Source: three-view drawing plus pictorial views. Frame: mm from the lowest corner of the part. A direction names the side the tool comes from. Coordinates: 2 decimals unless noted, no trailing zeros. Order: outer loops, then holes, each group sorted by start corner. A loop starts at its lowest first (then second) coordinate and runs counter-clockwise, first axis right, second up. Notation, with made-up numbers: (78.25, 55.5) - (136.25, 55.5) arc R23 cw to (136.25, 74.5) - close; hole circle Ø8 at (48, 16). An arc over 180 degrees is marked (long way). Use a Markdown table: item, result. Add a question column.
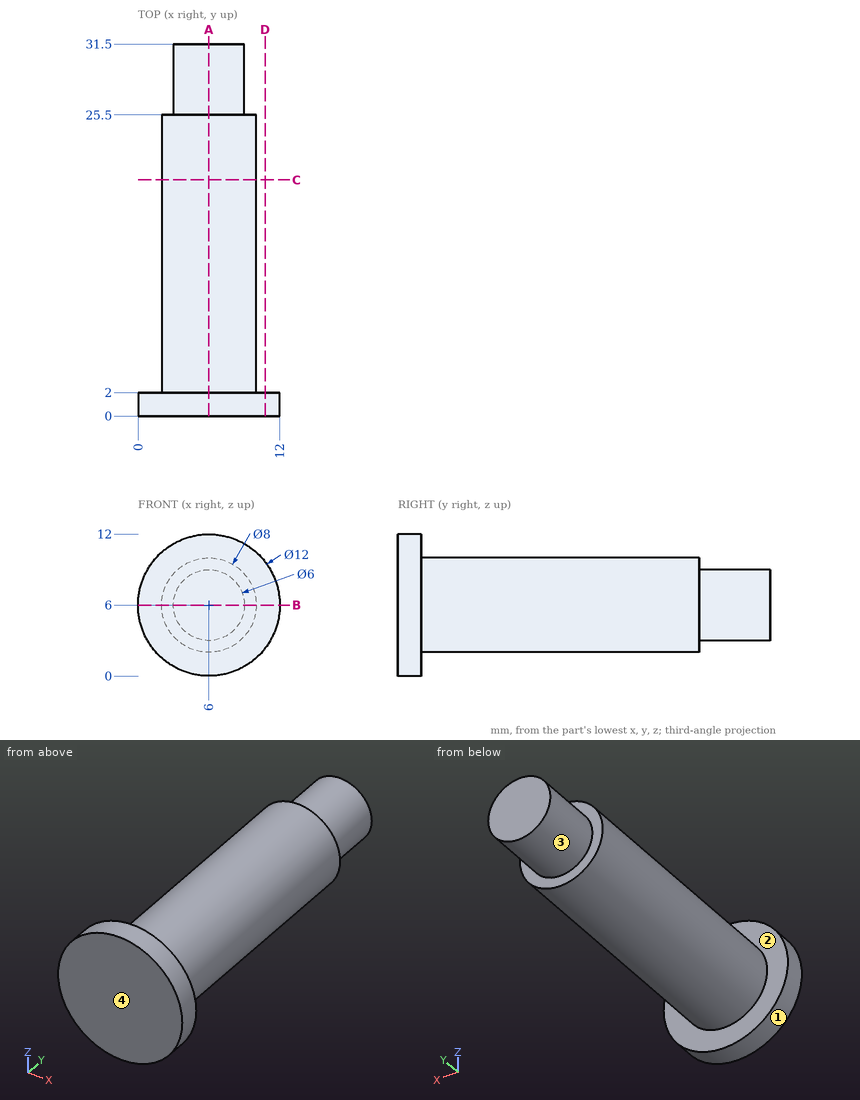
1) Draft query along Z for the marked faces 3 and 4. Return one class per face: pulls with the +Z half, pulls with the -Z half, needs draft (parallel to the pull), parting line crosses it, or undercut.
2) Section B-B (z = 6). Return loops of the section in (x, y), then the cut area to 3 significant figures.
3) Pin query (flat end, axial travel): pin 1 (1.5 mm diameter, centred on y = 20.5, z = 2, fed in from +X); pin 2 (6 mm diameter, centred on x = 9, y = 6, fed in from +Z); pin 3 (3 mm diameter, centred on x = 8.5, y = 8.5, fed in from -Z). Return the tip coordinate at first contact, or that it passes through.
4) Section D-D (x = 10.75). Return loops of the section in (y, z).
5) Ray query, line 1 along Y through (x, z) = (10.5, 6.25); line 2 along Y through (x, z) = (4, 9); line 3 along Z through (x, y) = (5.25, 20). Return the intervals inside material, ascending.
6) Section A-A (x = 6). Return loops of the section in (y, z), then the cut area to 3 significant figures.
7) Set-up query: the marked faces 1 and 2. Return all of +Z, -Z, +X, -X, +Y, -Y with unobstructed straight access to the full face (end or side cutting, diameter ignored); none if empty.
8) Section C-C (y = 20). Return loops of the section in (x, z).
Values follow:
| question | item | result |
|---|---|---|
| 1 | face 3 | parting line crosses it |
| 1 | face 4 | needs draft |
| 2 | outline | (0, 0) - (12, 0) - (12, 2) - (10, 2) - (10, 25.5) - (9, 25.5) - (9, 31.5) - (3, 31.5) - (3, 25.5) - (2, 25.5) - (2, 2) - (0, 2) - close |
| 2 | area | 248 mm² |
| 3 | pin 1 | stops at x = 8.33 |
| 3 | pin 2 | stops at z = 10 |
| 3 | pin 3 | stops at z = 2.13 |
| 4 | outline | (0, 2.33) - (2, 2.33) - (2, 9.67) - (0, 9.67) - close |
| 5 | line 1 | y = 0 to 2 |
| 5 | line 2 | y = 0 to 25.5 |
| 5 | line 3 | z = 2.07 to 9.93 |
| 6 | outline | (0, 0) - (2, 0) - (2, 2) - (25.5, 2) - (25.5, 3) - (31.5, 3) - (31.5, 9) - (25.5, 9) - (25.5, 10) - (2, 10) - (2, 12) - (0, 12) - close |
| 6 | area | 248 mm² |
| 7 | face 1 | +Y, -Y |
| 7 | face 2 | +Y |
| 8 | outline | circle Ø8 at (6, 6) |
